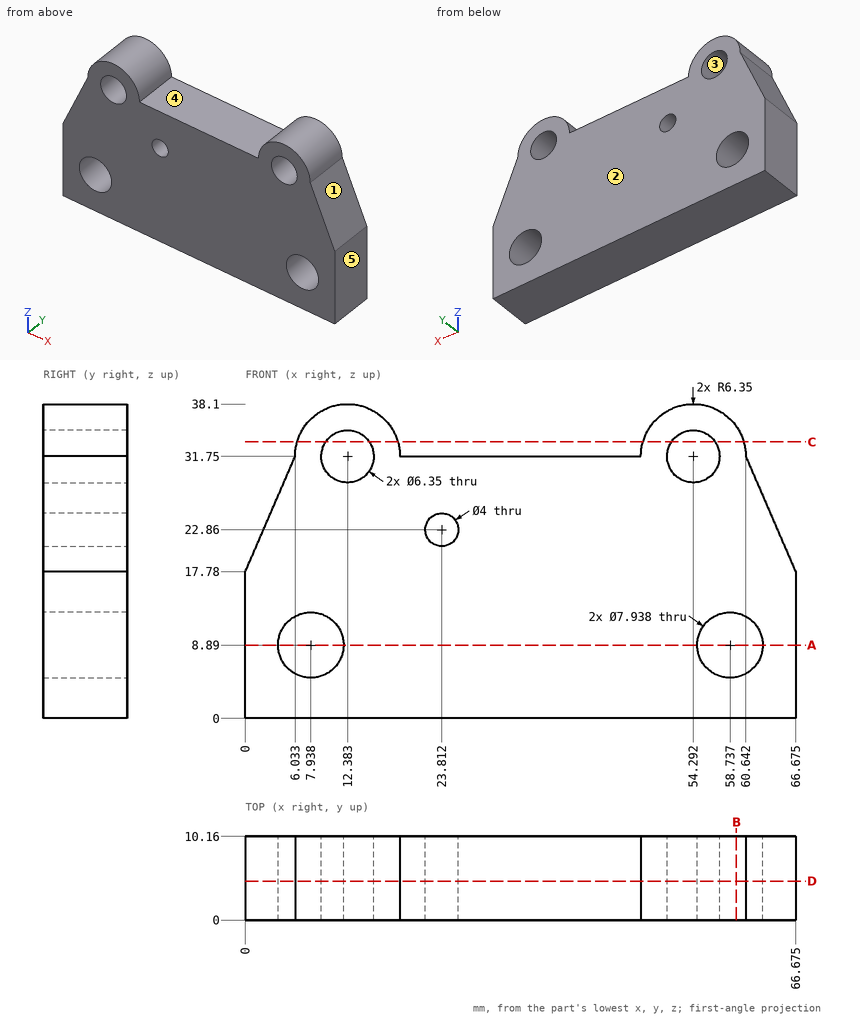
Geometry check sheet. Reference: drawing and pictorial views, mm from the part's lowest x, y, z. A direction names the side the tool comes from. Coordinates: 2 decimals unless noted, no trailing zeros. Order: outer loops, then holes, each group sorted by start corner. A loop starts at its lowest first (then second) coordinate and runs counter-clockwise, first axis right, second up. Notation, with made-up numbers: (-22, 80.5) -> (36, 80.5) arc R14 ccw to (36, 99.5) -> close; hole circle Ø1 at (-1.5, -9). An arc over 180 degrees is marked (long way). Put each result on its own line as item: value. Start each with the question number.
1) Cross-section at D-D (y = 4.75). State how many separate pieces and enclosed holes the cut face has, plus the area to 3 significant figures.
2) Cross-section at C-C (z = 33.5). Enter the section's corners in (x, y).
3) Material ranges on L1, parallel to X at y = 5.5, z = 8.89 (1 decimal); L2, parallel to X at y = 4, z = 32; L3, parallel to X at y = 3.25, z = 7.5 (1 decimal), recorded low to high.
4) Go/stop test with flat-tipped pins: pin 1 (1 mm diameter, centred on y = 2, z = 23.5, fed in from -X) (1 decimal); pin 2 (1 mm diameter, centred on x = 44.5, z = 13, fed in from -Y); pin 3 (1.5 mm diameter, centred on x = 36.5, y = 4, fed in from +Z); pin 4 (7 mm diameter, centred on x = 7.94, z = 8.89, fed in from +Y). Record where each tip stops, or that it passes through.
5) Cross-section at B-B (x = 59.5). Enter the section's corners in (y, z) (1 decimal).
6) Release check for a two-part mould opening along X. For the marked faces 1, 2 and 3 record: pulls with the +X half, pulls with the -X half, needs draft (parallel to the pull), parting line crosses it, or undercut.
7) Tool access check on the marked faces 4 and 5. Record the directions out of +Z, -Z, +X, -X, +Y, -Y that give a thin tool (end or side, any length) a straight path to the whole face; none if there is none.
8) Cross-section at A-A (z = 8.89). Enter the section's corners in (x, y) (1 decimal).
Geometry check:
1. separate pieces: 1
1. enclosed holes: 5
1. area: 1,980 mm^2
2. outline: (6.28, 0) -> (9.73, 0) -> (9.73, 10.16) -> (6.28, 10.16) -> close; (15.03, 0) -> (18.49, 0) -> (18.49, 10.16) -> (15.03, 10.16) -> close; (48.19, 0) -> (51.64, 0) -> (51.64, 10.16) -> (48.19, 10.16) -> close; (56.94, 0) -> (60.4, 0) -> (60.4, 10.16) -> (56.94, 10.16) -> close
3. L1: x = 0 to 4, 11.9 to 54.8, 62.7 to 66.7
3. L2: x = 6.04 to 9.22, 15.55 to 18.73, 47.95 to 51.13, 57.46 to 60.64
3. L3: x = 0 to 4.2, 11.7 to 55, 62.5 to 66.7
4. pin 1: stops at x = 2.3
4. pin 2: stops at y = 0
4. pin 3: stops at z = 31.75
4. pin 4: passes through
5. outline: (0, 0) -> (10.2, 0) -> (10.2, 5) -> (0, 5) -> close; (0, 12.8) -> (10.2, 12.8) -> (10.2, 35.4) -> (0, 35.4) -> close
6. face 1: pulls with the +X half
6. face 2: needs draft
6. face 3: undercut
7. face 4: +Z, +Y, -Y
7. face 5: +Z, -Z, +X, +Y, -Y
8. outline: (0, 0) -> (4, 0) -> (4, 10.2) -> (0, 10.2) -> close; (11.9, 0) -> (54.8, 0) -> (54.8, 10.2) -> (11.9, 10.2) -> close; (62.7, 0) -> (66.7, 0) -> (66.7, 10.2) -> (62.7, 10.2) -> close
